Design review of the part built by this model. Coordinates are the model's own, in mm. Face numbers are marked on the shaded views. A direction names the side the tool comes from. Round coordinates to 2 decimals unless told otherwise and drop trailing zeros. Order: outer loops, then holes, each group sorted by start corner. A loop starts at its lowest first (then second) coordinate and runs counter-clockwise, first axis right, second up.
from build123d import *

# Parameters (mm, degrees)
MODEL_R                 = 2.6
MODEL_R_2               = 4
SALIENTE_EXTRUIR1_DEPTH = 10
CROQUIS3_R              = 4
CORTAR_EXTRUIR1_DEPTH   = 5
CROQUIS4_R              = 7
CORTAR_EXTRUIR2_DEPTH   = 5


with BuildPart() as part:
    # Model → Saliente-Extruir1 (new body)
    with BuildSketch(Plane.XY):
        with BuildLine():
            Line((-15, 60), (15, 60))
            ThreePointArc((15, 60), (18.535533906, 58.535533906), (20, 55))
            Line((20, 55), (20, 26.442576537))
            ThreePointArc((20, 26.442576537), (33.154333863, 0), (20, -26.442576537))
            Line((20, -26.442576537), (20, -55))
            ThreePointArc((20, -55), (18.535533906, -58.535533906), (15, -60))
            Line((15, -60), (-15.011202946, -60))
            ThreePointArc((-15.011202946, -60), (-18.663093033, -58.415215776), (-20, -54.665479518))
            Line((-20, -54.665479518), (-20, -26.442576537))
            ThreePointArc((-20, -26.442576537), (-33.154333863, 0), (-20, 26.442576537))
            Line((-20, 26.442576537), (-20, 55))
            ThreePointArc((-20, 55), (-18.535533906, 58.535533906), (-15, 60))
        make_face()
        with Locations((-17.67766953, 17.677669526)):
            Circle(MODEL_R, mode=Mode.SUBTRACT)
        with Locations((-2e-09, 24.999999998)):
            Circle(MODEL_R, mode=Mode.SUBTRACT)
        with Locations((-24.999999998, -2e-09)):
            Circle(MODEL_R, mode=Mode.SUBTRACT)
        with Locations((17.677669526, 17.67766953)):
            Circle(MODEL_R, mode=Mode.SUBTRACT)
        with Locations((24.999999998, 2e-09)):
            Circle(MODEL_R, mode=Mode.SUBTRACT)
        with Locations((17.67766953, -17.677669526)):
            Circle(MODEL_R, mode=Mode.SUBTRACT)
        with Locations((2e-09, -24.999999998)):
            Circle(MODEL_R, mode=Mode.SUBTRACT)
        with Locations((-17.677669526, -17.67766953)):
            Circle(MODEL_R, mode=Mode.SUBTRACT)
        with Locations((0, 50)):
            Circle(MODEL_R_2, mode=Mode.SUBTRACT)
        with Locations(Location((0, -50, 0), (0, 0, 180))):
            Circle(MODEL_R_2, mode=Mode.SUBTRACT)
    extrude(amount=SALIENTE_EXTRUIR1_DEPTH)

    # Croquis3 → Cortar-Extruir1 (cut)
    with BuildSketch(Plane.XY.offset(10)):
        with Locations((24.999999998, 2e-09)):
            Circle(CROQUIS3_R)
        with Locations((17.67766953, -17.677669526)):
            Circle(CROQUIS3_R)
        with Locations((2e-09, -24.999999998)):
            Circle(CROQUIS3_R)
        with Locations((-17.677669526, -17.67766953)):
            Circle(CROQUIS3_R)
        with Locations((-24.999999998, -2e-09)):
            Circle(CROQUIS3_R)
        with Locations((-17.67766953, 17.677669526)):
            Circle(CROQUIS3_R)
        with Locations((-2e-09, 24.999999998)):
            Circle(CROQUIS3_R)
        with Locations((17.677669526, 17.67766953)):
            Circle(CROQUIS3_R)
    extrude(amount=-CORTAR_EXTRUIR1_DEPTH, mode=Mode.SUBTRACT)

    # Croquis4 → Cortar-Extruir2 (cut)
    with BuildSketch(Plane(origin=(0, 0, 0), x_dir=(-1, 0, 0), z_dir=(0, 0, -1))):
        with Locations((0, 50)):
            Circle(CROQUIS4_R)
        with Locations(Location((0, -50, 0), (0, 0, 180))):
            Circle(CROQUIS4_R)
    extrude(amount=-CORTAR_EXTRUIR2_DEPTH, mode=Mode.SUBTRACT)


solid = part.part
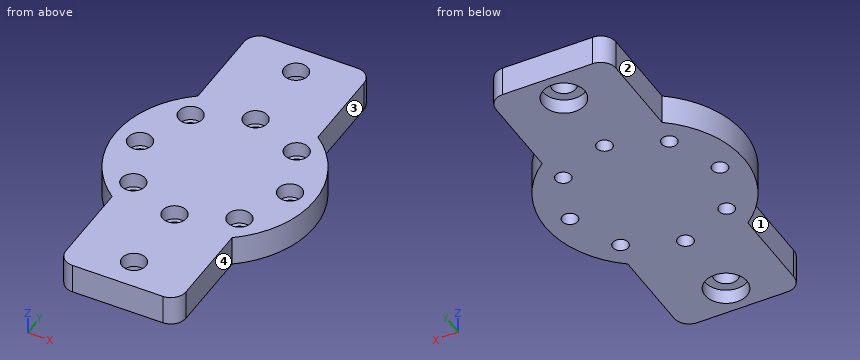
1) Take a section at B-B on y = 50. Give the boundary of the cut face in (x, z), plus the area to 3 significant figures.
Results:
outline: (-20, 0) - (-7, 0) - (-7, 5) - (-4, 5) - (-4, 10) - (-20, 10) - close; (4, 5) - (7, 5) - (7, 0) - (20, 0) - (20, 10) - (4, 10) - close
area: 290 mm2
2) Take a section at D-D on y = 35. Give the boundary of the cut face in (x, z).
Results:
outline: (-20, 0) - (20, 0) - (20, 10) - (-20, 10) - close
3) Take a section at A-A on y = 0. Give the boundary of the cut face in (x, z).
Results:
outline: (-33.15, 0) - (-27.6, 0) - (-27.6, 5) - (-29, 5) - (-29, 10) - (-33.15, 10) - close; (-22.4, 0) - (22.4, 0) - (22.4, 5) - (21, 5) - (21, 10) - (-21, 10) - (-21, 5) - (-22.4, 5) - close; (27.6, 0) - (33.15, 0) - (33.15, 10) - (29, 10) - (29, 5) - (27.6, 5) - close
4) Take a section at C-C on x = -25. Give the boundary of the cut face in (y, z).
Results:
outline: (-21.78, 0) - (-2.6, 0) - (-2.6, 5) - (-4, 5) - (-4, 10) - (-21.78, 10) - close; (2.6, 0) - (21.78, 0) - (21.78, 10) - (4, 10) - (4, 5) - (2.6, 5) - close
5) Clearance check with flat-ended pins moving along their axes: P1, Ø6, axis at x = -25, y = 0, coming from the +Z side; P2, Ø8.5, axis at x = 0, y = -50, coming from the -Z side; P3, Ø5, axis at y = -39.5, z = 3, coming from the -X side. State where each tip first meets the part, or that it passes through.
Results:
P1: stops at z = 5
P2: stops at z = 5
P3: stops at x = -20
6) To check wall thickness, follow line 1 along Y through (x, z) = (0, 1.4); line 2 along Y through (x, z) = (5.5, 4); line 3 along X through (y, z) = (-35, 4). State the ranges of each line that lie inside material, in increasing order.
Results:
line 1: y = -60 to -57, -43 to -27.6, -22.4 to 22.4, 27.6 to 43, 57 to 60
line 2: y = -60 to -54.33, -45.67 to 45.67, 54.33 to 60
line 3: x = -20 to 20
7) For the marked faces 1, 2, 3 and 4, list the 3-axis set-ups (+Z, -Z, +X, -X, +Y, -Y) from which the entire face can be reached by the end or side of a thin tool; tool diameter is ignored.
Results:
face 1: +Z, -Z, -X, -Y
face 2: +Z, -Z, -X, +Y
face 3: +Z, -Z, +X, +Y
face 4: +Z, -Z, +X, -Y
